Can you work these out from the drawing? Everything is in mm from the part's minimum corner. A direction names the side the tool comes from. Give positions to 0.01 mm unless a question says otherwise; leave off trailing zeros. Write each loop counter-clockwise with the first axis right and the second up, starting at its lowest first coordinate (ties: lowest second). Pieces come first, ordered by that corner, then holes. Notation, with made-up numbers: (59.5, 19.25) - (90.5, 19.25) arc R18 cw to (90.5, 26.25) - close; hole circle Ø6 at (-8, 76.5). An arc over 180 degrees is marked (long way). Use a Markdown table: item, result. Add a question column.
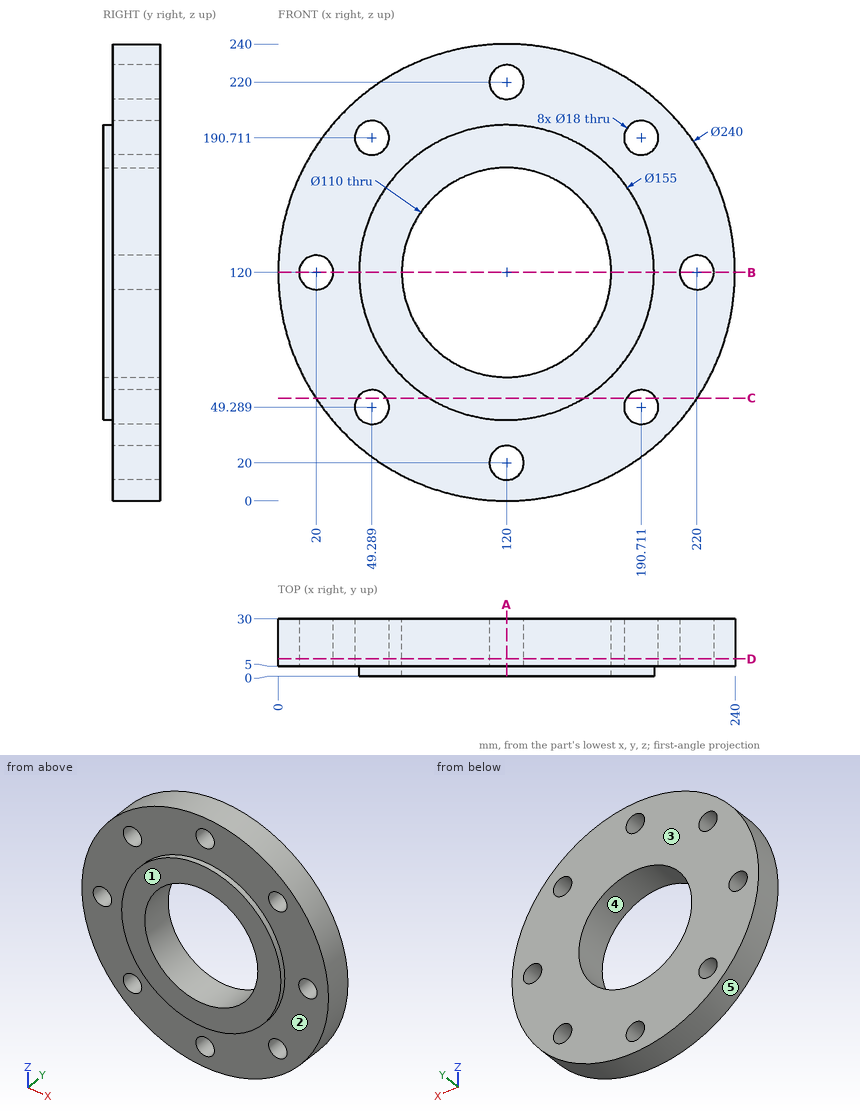
Q1. If we mould it in two halves opening along Z, with no side actions, what happens to the marked faces 3, 4 and 5? For each: released by +Z, released by -Z, zero draft, split by the parting line, or undercut.
Q2. On a 3-axis mill with a long thin cutter (end or side, diameter ignored), from which of +Z, -Z, +X, -X, +Y, -Y can I reach the whole of each face in a straight line? I mean the marked faces 1 and 2. Say none if no direction works.
Q3. Suppose I cut it at D-D (y = 9). Give the number of separate pieces and of enclosed holes in the cut face, and give its area (3 significant figures).
Q4. I'm going to push flat-ended pins straight in: P1, Ø14.5, axis at x = 190.71, z = 190.71, coming from the +Y side; P2, Ø12, axis at y = 16, z = 88, coming from the +X side; P3, Ø8, axis at x = 178.5, y = 8, coming from the +Z side; P4, Ø5, axis at y = 25.5, z = 45.5, coming from the -X side. Where does each tip first touch, or does it pass through?
Q5. Suppose I cut it at B-B (z = 120). Please give me the cut outline in (x, y).
Q6. Suppose I cut it at C-C (z = 54). Please give me the cut outline in (x, y), and give its area (3 significant figures).
Q7. Suppose I cut it at A-A (x = 120). Please give me the cut outline in (y, z), and give its area (4 significant figures).
Q8. If I drill on probe 1 along Z at (x, y) = (120, 19.5); probe 2 along Z at (x, y) = (43, 23); probe 3 along Y at (x, z) = (64, 32), over which ranges is the centre line in solid material (lowest first)? Write a range as [from, to].
Derived:
| question | item | result |
|---|---|---|
| 1 | face 3 | zero draft |
| 1 | face 4 | undercut |
| 1 | face 5 | split by the parting line |
| 2 | face 1 | +Z, -Z, +X, -X, -Y |
| 2 | face 2 | -Y |
| 3 | separate pieces | 1 |
| 3 | enclosed holes | 9 |
| 3 | area | 33,700 mm² |
| 4 | P1 | through |
| 4 | P2 | x = 237.15 |
| 4 | P3 | z = 226.91 |
| 4 | P4 | x = 24 |
| 5 | outline | (0, 5) - (11, 5) - (11, 30) - (0, 30) - close; (29, 5) - (42.5, 5) - (42.5, 0) - (65, 0) - (65, 30) - (29, 30) - close; (175, 0) - (197.5, 0) - (197.5, 5) - (211, 5) - (211, 30) - (175, 30) - close; (229, 5) - (240, 5) - (240, 30) - (229, 30) - close |
| 6 | outline | (19.78, 5) - (41.62, 5) - (41.62, 30) - (19.78, 30) - close; (56.96, 5) - (79.38, 5) - (79.38, 0) - (160.62, 0) - (160.62, 5) - (183.04, 5) - (183.04, 30) - (56.96, 30) - close; (198.38, 5) - (220.22, 5) - (220.22, 30) - (198.38, 30) - close |
| 6 | area | 4,650 mm² |
| 7 | outline | (0, 42.5) - (5, 42.5) - (5, 29) - (30, 29) - (30, 65) - (0, 65) - close; (0, 175) - (30, 175) - (30, 211) - (5, 211) - (5, 197.5) - (0, 197.5) - close; (5, 0) - (30, 0) - (30, 11) - (5, 11) - close; (5, 229) - (30, 229) - (30, 240) - (5, 240) - close |
| 7 | area | 2,575 mm² |
| 8 | probe 1 | [0, 11], [29, 65], [175, 211], [229, 240] |
| 8 | probe 2 | [27.96, 42.85], [55.73, 184.27], [197.15, 212.04] |
| 8 | probe 3 | [5, 30] |
